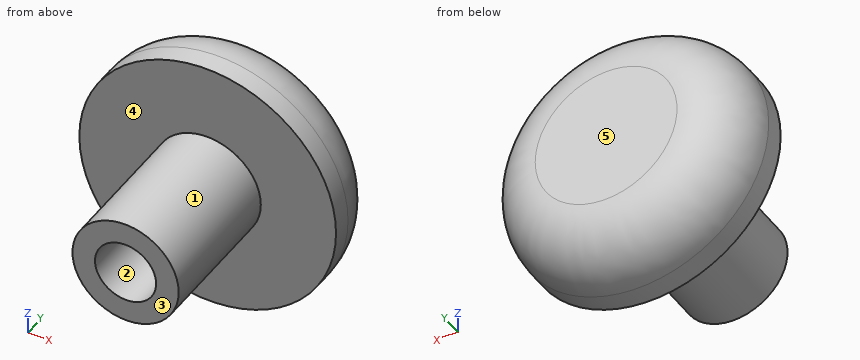
from build123d import *

# Parameters (mm, degrees)
FILLET1_R                 = 2.54
F_6_32_TAPPED_HOLE1_D     = 2.7051
F_6_32_TAPPED_HOLE1_DEPTH = 5.8928
F_6_32_TAPPED_HOLE1_TIP   = 0.81269403


with BuildPart() as part:
    # Sketch1 → Revolve1 (revolve)
    with BuildSketch(Plane.XY, mode=Mode.PRIVATE) as revolve1_sk:
        Polygon((0, 0), (-5.6769, 0), (-5.6769, -3.429), (-2.3495, -3.429), (-2.3495, -9.525), (0, -9.525), align=None)
    revolve(revolve1_sk.sketch.rotate(Axis((0, -9.525, 0), (0, 1, 0)), 180), axis=Axis((0, -9.525, 0), (0, 1, 0)))

    # Fillet1
    fillet1_edges = [part.edges().sort_by_distance(p)[0] for p in [
        (-5.6769, 0, 0),
    ]]
    fillet(fillet1_edges, radius=FILLET1_R)

    # #6-32 Tapped Hole1
    with Locations(Plane.XZ.offset(9.525)):
        with Locations((0, 0)):
            Hole(F_6_32_TAPPED_HOLE1_D / 2, depth=F_6_32_TAPPED_HOLE1_DEPTH)
            with Locations((0, 0, -(F_6_32_TAPPED_HOLE1_DEPTH + F_6_32_TAPPED_HOLE1_TIP / 2))):  # 118° drill point
                Cone(0, F_6_32_TAPPED_HOLE1_D / 2, F_6_32_TAPPED_HOLE1_TIP, mode=Mode.SUBTRACT)


solid = part.part
Can you work these out from the model? Positions are in its coordinate system, mm. Face numbers are marked on the shaded views. A direction names the side the tool comes from. Coordinates: 2 decimals unless noted, no trailing zeros. Write each loop counter-clockwise with the first axis right and the second up, starting at its lowest first coordinate (ties: lowest second). Pieces come first, ordered by that corner, then holes.
Q1. For P1, Ø1, axis at y = -5.5, z = -4, coming from the -X side; P2, Ø1.5, axis at x = -3, z = -2, coming from the -Y side; P3, Ø2, axis at x = -2, z = 4, coming from the +Y side; P4, Ø5, axis at x = 3, y = -1, coming from the +Z side, each with a flat end and sliding along its axis, tell me the tip position at first contact or that it passes through.
Results found:
P1: passes through
P2: stops at y = -3.43
P3: stops at y = -0.02
P4: stops at z = 5.6
Q2. Which directions (+Z, -Z, +X, -X, +Y, -Y) give clear straight access to the entire face, cutting with the end or side of a thin tool? Please do the marked faces 4 and 5.
Results found:
face 4: -Y
face 5: +Z, -Z, +X, -X, +Y
Q3. Imagine slicing it at A-A, the plane y = -8. List the corners of the cut face in (x, z) for me.
Results found:
outline: circle Ø4.7 at (0, 0); hole circle Ø2.71 at (0, 0)
Q4. Imagine slicing it at B-B, the plane y = -3.25. List the corners of the cut face in (x, z) for me, plus the area to 3 significant figures.
Results found:
outline: circle Ø11.35 at (0, 0); hole circle Ø1.43 at (0, 0)
area: 99.6 mm2
Q5. Please list where these lines run through material, in increasing order: L1, parallel to Z at x = 0, y = -5.45; L2, parallel to Z at x = 1, y = -7.5; L3, parallel to Y at x = 1.5, z = -2.
Results found:
L1: z = -2.35 to -1.35, 1.35 to 2.35
L2: z = -2.13 to -0.91, 0.91 to 2.13
L3: y = -3.43 to 0
Q6. If we mould it in two halves opening along X, with no side actions, what happens to the marked faces 1, 2 and 3? For each: +X half, -X half, draft (parallel to the pull), parting line (faces both ways), or undercut.
Results found:
face 1: parting line
face 2: undercut
face 3: draft
